```python
from build123d import *

# Parameters (mm, degrees)
BOSS_EXTRUDE1_DEPTH = 60
FILLET1_R           = 1


with BuildPart() as part:
    # Sketch2 → Boss-Extrude1 (new body)
    with BuildSketch(Plane(origin=(0, 0, 0), x_dir=(-1, 0, 0), z_dir=(0, 1, 0))):
        Polygon((0.743842872, 43.599274051), (1.650150659, 44.021892313), (0.382295874, 46.740815674), (-19.647106212, 37.400952093), (-13.647106212, -5), (16.726783574, -5), (18.726783574, 7.400934848), (17.794168258, 9.400934848), (16.887860471, 8.978316586), (17.310478732, 8.072008799), (0, 0), (-16.989254122, 36.433573039), (0.32122461, 44.505581838), align=None)
    extrude(amount=BOSS_EXTRUDE1_DEPTH)

    # Fillet1
    fillet1_edges = [part.edges().sort_by_distance(p)[0] for p in [
        (-18.726783574, 30, 7.400934848),
        (19.647106212, 30, 37.400952093),
        (-0.382295874, 30, 46.740815674),
    ]]
    fillet(fillet1_edges, radius=FILLET1_R)


solid = part.part
```
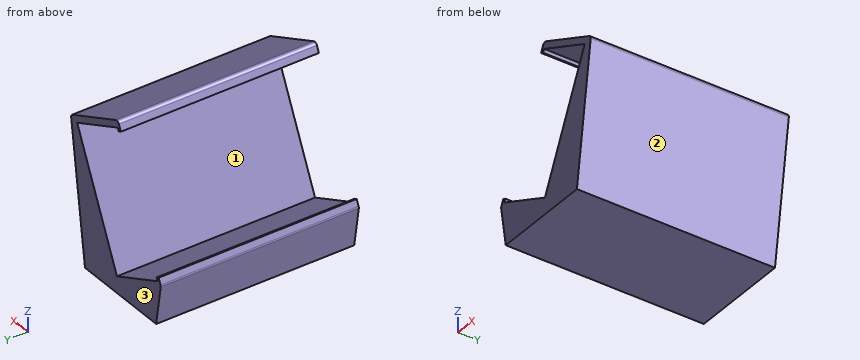
For this review, take the finished solid that the model builds, in its own axes (mm). Face numbers are marked on the shaded views. Give positions to 0.01 mm unless a question says otherwise; leave off trailing zeros. Write each loop counter-clockwise with the first axis right and the second up, starting at its lowest first coordinate (ties: lowest second). Pieces come first, ordered by that corner, then holes. Notation, with made-up numbers: M -27,59.5 L 24,59.5 A24 ccw 24,90.5 Z; hole C 61,60.25 d7. An arc over 180 degrees is marked long. One line per item, written item: value.
1) Take a section at C-C, the plane x = 12. Write out the cut boundary in (y, z), then the cut area to 3 significant figures.
Results are:
outline: M 0,-5 L 60,-5 L 60,25.73 L 0,25.73 Z; M 0,38.76 L 60,38.76 L 60,40.97 L 0,40.97 Z
area: 1,980 mm²
2) Take a section at B-B, the plane y = 30. Write out the cut boundary in (x, z).
Results are:
outline: M -18.68,7.1 L -16.73,-5 L 13.65,-5 L 19.54,36.67 A1 ccw 18.98,37.71 L 0.52,46.32 A1 ccw -0.8,45.83 L -1.65,44.02 L -0.74,43.6 L -0.32,44.51 L 16.99,36.43 L 0,0 L -17.31,8.07 L -16.89,8.98 L -17.79,9.4 L -18.6,7.68 A1 ccw Z
3) Take a section at A-A, the plane x = 7.5. Write out the cut boundary in (y, z).
Results are:
outline: M 0,-5 L 60,-5 L 60,16.08 L 0,16.08 Z; M 0,40.86 L 60,40.86 L 60,43.07 L 0,43.07 Z
4) The part is to be moulded in two halves that separate along X. For the marked faces 1, 2 and 3, say which applies: +X half, -X half, draft (parallel to the pull), parting line (faces both ways), or undercut.
Results are:
face 1: undercut
face 2: +X half
face 3: draft
5) For line 1 (Z direction, x = -0.5, y = 4); line 2 (Z direction, x = 13.5, y = 25); line 3 (X direction, y = 5.5, z = 13), list the stretches that pass through material, from the lowest coordinate up. Write a range as from..to.
Results are:
line 1: z = -5..0.23, 44.12..46.21
line 2: z = -5..28.95, 38.06..40.27
line 3: x = 6.06..16.19
6) Take a section at D-D, the plane z = 34.5. Write out the cut boundary in (x, y).
Results are:
outline: M 16.09,0 L 19.24,0 L 19.24,60 L 16.09,60 Z
7) For P1, Ø10, axis at y = 33.5, z = 29, coming from the -X side; P2, Ø8, axis at y = 44, z = 27.5, coming from the +X side; P3, Ø1, axis at y = 53.5, z = 13.5, coming from the -X side; P4, Ø12, axis at x = -2.5, z = 33, coming from the +Y side, all flat-tipped, find the tip position at first contact; note any pin that passes through.
Results are:
P1: stops at x = 11.19
P2: stops at x = 18.81
P3: stops at x = 6.06
P4: passes through
